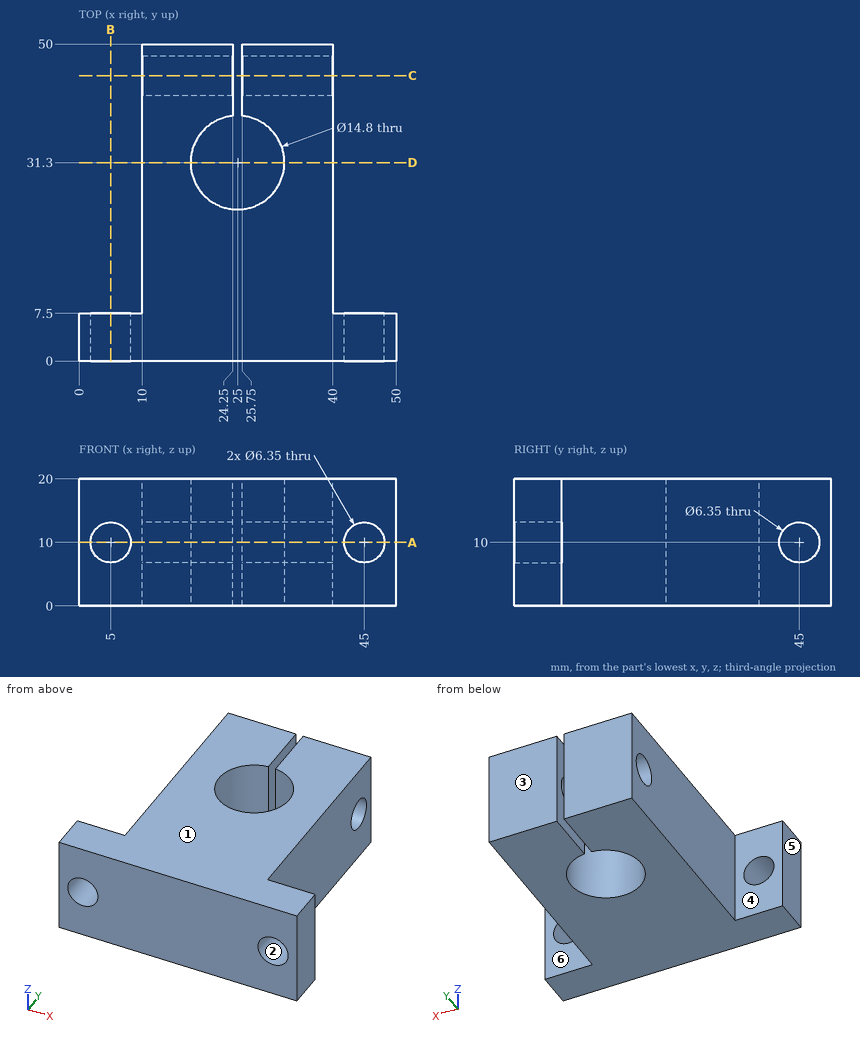
Job drawing, mm, ordinate dimensions from the low corner. One solid piece. A direction names the side the tool comes from. Coordinates: 2 decimals unless noted, no trailing zeros. Write each loop counter-clockwise with the first axis right and the second up, starting at its lowest first coordinate (ties: lowest second). Pieces come first, ordered by that corner, then holes.
Item 1: Slice it at C-C (y = 45). Write the cut outline in (x, z) (3 decimals).
Item 2: Pin check, flat tips, straight feed: pin 1 (5.5 mm diameter, centred on y = 46, z = 8, fed in from +X); pin 2 (5 mm diameter, centred on y = 45, z = 10, fed in from -X); pin 3 (10 mm diameter, centred on x = 45, z = 10, fed in from -Y); pin 4 (1.5 mm diameter, centred on y = 10.5, z = 11.5, fed in from -X). Stop position of each tip, or through.
Item 3: Which spindle directions (+Z, -Z, +X, -X, +Y, -Y) get a long thin tool onto all of the face, cutting with end or side? Do the marked faces 4, 5 and 6. Say none if no direction does.
Item 4: Slice it at D-D (y = 31.3). Write the cut outline in (x, z), and give its area (3 significant figures).
Item 5: Probe line 1 (X direction, y = 6, z = 10.25); line 2 (Z direction, x = 28.75, y = 45) (3 decimals); line 3 (X direction, y = 40.5, z = 16.25). List the from-to ranges inside material, lowest first.
Item 6: Slice it at A-A (z = 10). Write the cut outline in (x, y) (3 decimals), and give its area (3 significant figures).
Item 7: Slice it at B-B (x = 5). Write the cut outline in (y, z) (3 decimals).
Item 8: Mould opens along Z. For the marked faces 1, 2 and 3 say: released by +Z, released by -Z, zero draft, split by the parting line, or undercut.
Results found:
1. outline: (10, 0) - (24.25, 0) - (24.25, 6.825) - (10, 6.825) - close; (10, 13.175) - (24.25, 13.175) - (24.25, 20) - (10, 20) - close; (25.75, 0) - (40, 0) - (40, 6.825) - (25.75, 6.825) - close; (25.75, 13.175) - (40, 13.175) - (40, 20) - (25.75, 20) - close
2. pin 1: stops at x = 40
2. pin 2: passes through
2. pin 3: stops at y = 0
2. pin 4: stops at x = 10
3. face 4: +Z, -Z, -X, +Y
3. face 5: +Z, -Z, -X, +Y, -Y
3. face 6: +Z, -Z, +X, +Y
4. outline: (10, 0) - (17.6, 0) - (17.6, 20) - (10, 20) - close; (32.4, 0) - (40, 0) - (40, 20) - (32.4, 20) - close
4. area: 304 mm2
5. line 1: x = 0 to 1.83, 8.17 to 41.83, 48.17 to 50
5. line 2: z = 0 to 6.825, 13.175 to 20
5. line 3: x = 10 to 24.25, 25.75 to 40
6. outline: (0, 0) - (1.825, 0) - (1.825, 7.5) - (0, 7.5) - close; (8.175, 0) - (41.825, 0) - (41.825, 7.5) - (40, 7.5) - (40, 41.825) - (25.75, 41.825) - (25.75, 38.662) arc R7.4 cw (long way) to (24.25, 38.662) - (24.25, 41.825) - (10, 41.825) - (10, 7.5) - (8.175, 7.5) - close; (10, 48.175) - (24.25, 48.175) - (24.25, 50) - (10, 50) - close; (25.75, 48.175) - (40, 48.175) - (40, 50) - (25.75, 50) - close; (48.175, 0) - (50, 0) - (50, 7.5) - (48.175, 7.5) - close
6. area: 1,180 mm2
7. outline: (0, 0) - (7.5, 0) - (7.5, 6.825) - (0, 6.825) - close; (0, 13.175) - (7.5, 13.175) - (7.5, 20) - (0, 20) - close
8. face 1: released by +Z
8. face 2: undercut
8. face 3: zero draft
